Answer from the drawing. Dimensions are ordinates in mm from the lowest x, y and z of the part. A direction names the side the tool comes from. Coordinates: 2 decimals unless noted, no trailing zeros. Write each loop counter-clockwise with the first axis right and the second up, starting at its lowest first coordinate (ties: lowest second). Pieces come first, ordered by that corner, then holes. Notation, with made-up numbers: (-3.75, 53) -> (16.25, 53) arc R20 cw to (16.25, 61) -> close; hole circle Ø5 at (79, 76.5). An arc over 180 degrees is marked (long way). Answer as a JSON object with one key per item and string values. Group by question number.
(1) Which of the six approach directions +Z, -Z, +X, -X, +Y, -Y give full straight-line access (tool end or side, diameter ignored) to the marked faces 1 and 2?
(2) Find section D-D (z = 15). Give the vertices of the cut face in (x, y).
(3) For a pull along Z with two mould halves and no side action, classify the marked faces 3, 4 and 5 as +Z half, -Z half, draft (parallel to the pull), parting line (faces both ways), or undercut.
(4) Find section A-A (x = 11). Give the vertices of the cut face in (y, z).
(5) Find section B-B (z = 11). Give the vertices of the cut face in (x, y), then the cut area to 3 significant figures.
(6) Find section C-C (y = 1.75). Give the vertices of the cut face in (x, z), then the cut area to 3 significant figures.
(7) Straight lines are drawn through the part: L1, parallel to Z at x = 11, y = 8.95; L2, parallel to Z at x = 11, y = 5.75; L3, parallel to Y at x = 16, z = 13. For each, find the intervals that lie inside material, in ascending order.
(8) Flat-ended cylindrical pins translate along their axes: P1, Ø5.5, axis at x = 11.5, z = 13.5, coming from the -Y side; P2, Ø3, axis at x = 12, y = 1.5, coming from the -Z side; P3, Ø4, axis at x = 3.5, y = 3, coming from the +Z side; P4, Ø5, axis at y = 4, z = 5.5, coming from the +X side. Find the tip coordinate at first contact, or state that the pin passes through.
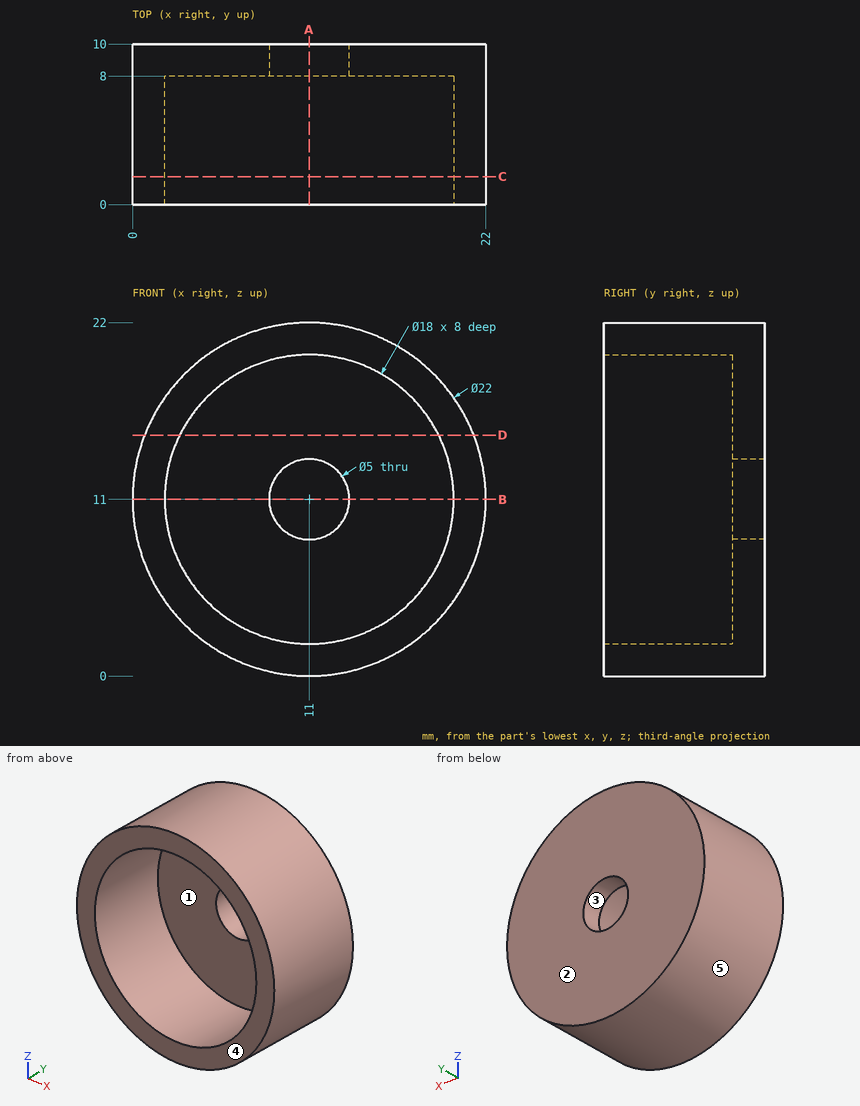
Results below:
{
 "1": {"face 1": "-Y", "face 2": "+Z, -Z, +X, -X, +Y"},
 "2": {"outline": "(0.75, 0) -> (2.94, 0) -> (2.94, 8) -> (19.06, 8) -> (19.06, 0) -> (21.25, 0) -> (21.25, 10) -> (0.75, 10) -> close"},
 "3": {"face 3": "undercut", "face 4": "draft", "face 5": "parting line"},
 "4": {"outline": "(0, 0) -> (10, 0) -> (10, 8.5) -> (8, 8.5) -> (8, 2) -> (0, 2) -> close; (0, 20) -> (8, 20) -> (8, 13.5) -> (10, 13.5) -> (10, 22) -> (0, 22) -> close"},
 "5": {"outline": "(0, 0) -> (2, 0) -> (2, 8) -> (8.5, 8) -> (8.5, 10) -> (0, 10) -> close; (13.5, 8) -> (20, 8) -> (20, 0) -> (22, 0) -> (22, 10) -> (13.5, 10) -> close", "area": "66.0 mm2"},
 "6": {"outline": "circle Ø22 at (11, 11); hole circle Ø18 at (11, 11)", "area": "126 mm2"},
 "7": {"L1": "z = 0 to 8.5, 13.5 to 22", "L2": "z = 0 to 2, 20 to 22", "L3": "y = 8 to 10"},
 "8": {"P1": "stops at y = 8", "P2": "stops at z = 0", "P3": "stops at z = 20.53", "P4": "stops at x = 21.58"}
}
